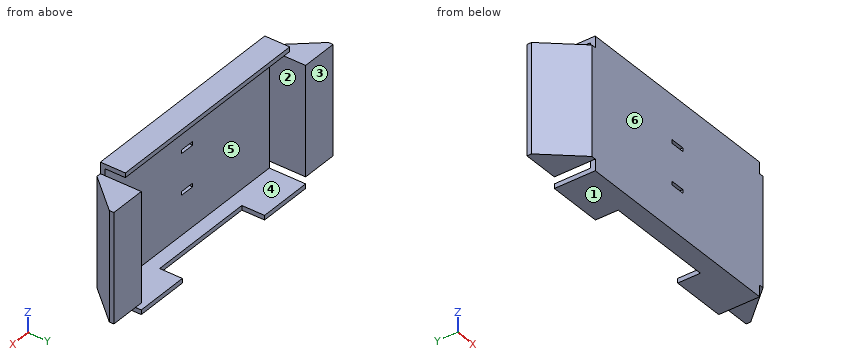
Autodesk Fusion 360 part; units mm, degrees
sketch "Sketch4" plane through (0, 0, 0) normal (0, 1, 0) x (1, 0, 0)
  line L0 (0, 0) -> (152.4, 0)
  line L1 (152.4, 0) -> (152.4, 85.725)
  line L2 (152.4, 85.725) -> (0, 85.725)
  line L3 (0, 85.725) -> (0, 0)
  dimension "d16" = 152.4
  dimension "d17" = 85.725
extrude "Extrude4" add sketch "Sketch4" along normal blind 3.175
sketch "Sketch5" plane through (0, 0, 0) normal (0, 0, 1) x (1, 0, 0)
  line L0 (0, 0) -> (152.4, 0)
  line L1 (152.4, 0) -> (152.4, 3.175)
  line L2 (152.4, 3.175) -> (0, 3.175)
  line L3 (0, 3.175) -> (0, 0)
  line L4 (0, 3.175) -> (152.4, 3.175)
  line L5 (0, 0) -> (152.4, 0)
  line L6 (0, 0) -> (0, 3.175)
  line L7 (152.4, 0) -> (152.4, 3.175)
  line L8 (152.4, 0) -> (152.4, 17.4625)
  line L9 (0, 0) -> (0, 17.4625)
  line L10 (0, 17.4625) -> (152.4, 17.4625)
  dimension "d20" = 17.4625
  dimension "d21" = 17.4625
extrude "Extrude5" add sketch "Sketch5" along normal blind 3.175
sketch "Sketch6" plane through (0, 0, -85.725) normal (0, 0, -1) x (-1, 0, 0)
  line L0 (-152.4, 0) -> (0, 0)
  line L1 (0, 0) -> (0, 3.175)
  line L2 (0, 3.175) -> (-152.4, 3.175)
  line L3 (-152.4, 3.175) -> (-152.4, 0)
  line L4 (-152.4, 3.175) -> (0, 3.175)
  line L5 (-152.4, 0) -> (-152.4, 3.175)
  line L6 (-152.4, 0) -> (0, 0)
  line L7 (0, 0) -> (0, 3.175)
  line L8 (0, 0) -> (0, 28.575)
  line L9 (0, 28.575) -> (-38.1, 28.575)
  line L10 (-38.1, 28.575) -> (-38.1, 12.7)
  line L11 (-38.1, 12.7) -> (-114.3, 12.7)
  line L12 (-114.3, 12.7) -> (-114.3, 28.575)
  line L13 (-114.3, 28.575) -> (-152.4, 28.575)
  line L14 (-152.4, 28.575) -> (-152.4, 0)
  dimension "d24" = 28.575
  dimension "d25" = 38.1
  dimension "d26" = 15.875
  dimension "d27" = 76.2
  dimension "d28" = 15.875
  dimension "d29" = 38.1
extrude "Extrude6" add sketch "Sketch6" along normal blind 3.175
sketch "Sketch7" plane through (0, 0, 0) normal (-1, 0, 0) x (0, 0, 1)
  line L0 (-88.9, 0) -> (3.175, 0)
  line L1 (3.175, 0) -> (3.175, 17.4625)
  line L2 (3.175, 17.4625) -> (0, 17.4625)
  line L3 (0, 17.4625) -> (0, 3.175)
  line L4 (0, 3.175) -> (-85.725, 3.175)
  line L5 (-85.725, 3.175) -> (-85.725, 28.575)
  line L6 (-85.725, 28.575) -> (-88.9, 28.575)
  line L7 (-88.9, 28.575) -> (-88.9, 0)
  line L8 (-85.725, 3.175) -> (-85.725, 28.575)
  line L9 (-85.725, 28.575) -> (-88.9, 28.575)
  line L10 (-88.9, 0) -> (-88.9, 28.575)
  line L11 (-85.725, 3.175) -> (0, 3.175)
  line L12 (0, 3.175) -> (0, 17.4625)
  line L13 (0, 17.4625) -> (3.175, 17.4625)
  line L14 (3.175, 17.4625) -> (3.175, 0)
  line L15 (-88.9, 0) -> (3.175, 0)
  line L16 (-85.725, 3.175) -> (-80.9625, 3.175) construction
  line L17 (0, 3.175) -> (-4.7625, 3.175) construction
  line L18 (-80.9625, 0) -> (-80.9625, 28.575)
  line L19 (-4.7625, 0) -> (-4.7625, 28.575)
  line L20 (-80.9625, 28.575) -> (-4.7625, 28.575)
  dimension "d35" = 4.7625
  dimension "d36" = 4.7625
  dimension "d37" = 28.575
  dimension "d38" = 28.575
  dimension "d39" = 76.2
extrude "Extrude7" add sketch "Sketch7" along normal blind 3.175 contours L0 L4 L11 L15 L18 L19 | L4 L11 L18 L19 L20
sketch "Sketch8" plane through (0, 28.575, 0) normal (0, 1, 0) x (-1, 0, 0)
  line L0 (0, -4.7625) -> (0, -80.9625)
  line L1 (0, -80.9625) -> (3.175, -80.9625)
  line L2 (3.175, -80.9625) -> (3.175, -4.7625)
  line L3 (3.175, -4.7625) -> (0, -4.7625)
  line L4 (0, -80.9625) -> (3.175, -80.9625)
  line L5 (0, -80.9625) -> (0, -4.7625)
  line L6 (3.175, -4.7625) -> (3.175, -80.9625)
  line L7 (0, -4.7625) -> (3.175, -4.7625)
  line L8 (0, -4.7625) -> (25.4, -4.7625)
  line L9 (0, -80.9625) -> (25.4, -80.9625)
  line L10 (25.4, -80.9625) -> (25.4, -4.7625)
  dimension "d42" = 25.4
  dimension "d43" = 25.4
  dimension "d44" = 76.2
extrude "Extrude9" add sketch "Sketch8" against normal blind 3.175 contours L2 L6 L8 L9 L10
ref_plane "WorkPlane1" through (76.2, 14.2875, -42.8625) normal (1, 0, 0) x (0, 0, -1)
mirror "Mirror1" about plane through (76.2, 14.2875, -42.8625) normal (1, 0, 0) of "Extrude7"
mirror "Mirror3" about plane through (76.2, 14.2875, -42.8625) normal (1, 0, 0) of "Extrude9"
sketch "Sketch9" plane through (0, 0, -80.9625) normal (0, 0, -1) x (-1, 0, 0)
  line L0 (-152.4, 0) -> (-152.4, 3.175)
  line L1 (-152.4, 3.175) -> (-152.4, 28.575)
  line L2 (-152.4, 28.575) -> (-177.8, 28.575)
  line L3 (-177.8, 28.575) -> (-177.8, 25.4)
  line L4 (-177.8, 25.4) -> (-155.575, 25.4)
  line L5 (-155.575, 25.4) -> (-155.575, 0)
  line L6 (-155.575, 0) -> (-152.4, 0)
  line L7 (-177.8, 25.4) -> (-155.575, 0)
extrude "Extrude10" add sketch "Sketch9" against normal up to surface (76.2 mm away) contours L4 L5 L7
mirror "Mirror4" about plane through (76.2, 14.2875, -42.8625) normal (1, 0, 0) of "Extrude10"
sketch "Sketch10" plane through (0, 3.175, 0) normal (0, 1, 0) x (-1, 0, 0)
  line L0 (0, -85.725) -> (0, -80.9625)
  line L1 (0, -80.9625) -> (0, -4.7625)
  line L2 (0, -4.7625) -> (0, 0)
  line L3 (0, 0) -> (-152.4, 0)
  line L4 (-152.4, 0) -> (-152.4, -4.7625)
  line L5 (-152.4, -4.7625) -> (-152.4, -80.9625)
  line L6 (-152.4, -80.9625) -> (-152.4, -85.725)
  line L7 (-152.4, -85.725) -> (0, -85.725)
  line L8 (0, -80.9625) -> (0, -4.7625)
  line L9 (-152.4, -85.725) -> (0, -85.725)
  line L10 (0, -85.725) -> (0, -80.9625)
  line L11 (0, -4.7625) -> (0, 0)
  line L12 (0, 0) -> (-152.4, 0)
  line L13 (-152.4, -4.7625) -> (-152.4, -80.9625)
  line L14 (-152.4, -80.9625) -> (-152.4, -85.725)
  line L15 (-152.4, 0) -> (-152.4, -4.7625)
  line L16 (0, -85.725) -> (-152.4, 0) construction
  line L17 (-152.4, -85.725) -> (0, 0) construction
  line L18 (-76.2, -42.8625) -> (-88.2955, -42.8625) construction
  line L19 (-76.2, -42.8625) -> (-64.1096, -42.8625) construction
  line L20 (-64.1096, -42.8625) -> (-64.1096, -58.3692) construction
  line L21 (-64.1096, -42.8625) -> (-64.1096, -27.3558) construction
  line L22 (-64.1096, -58.3692) -> (-88.2904, -58.3692) construction
  line L23 (-64.1096, -27.3558) -> (-88.2904, -27.3558) construction
  line L24 (-88.2904, -58.3692) -> (-88.2904, -27.3558) construction
  line L25 (-64.1096, -58.3692) -> (-71.12, -58.3692) construction
  line L26 (-88.2904, -58.3692) -> (-81.28, -58.3692) construction
  line L27 (-64.1096, -27.3558) -> (-71.12, -27.3558) construction
  line L28 (-71.12, -58.3692) -> (-71.12, -55.8292)
  line L29 (-71.12, -55.8292) -> (-81.28, -55.8292)
  line L30 (-81.28, -55.8292) -> (-81.28, -58.3692)
  line L31 (-71.12, -58.3692) -> (-81.28, -58.3692)
  line L32 (-71.12, -27.3558) -> (-71.12, -29.8958)
  line L33 (-71.12, -29.8958) -> (-81.28, -29.8958)
  line L34 (-81.28, -29.8958) -> (-81.28, -27.3558)
  line L35 (-64.1096, -27.3558) -> (-88.2904, -27.3558) construction
  line L36 (-71.12, -27.3558) -> (-81.28, -27.3558)
  point P0 (-152.4, -85.725)
  dimension "d61" = 15.5067
  dimension "d62" = 15.5067
  dimension "d63" = 24.1808
  dimension "d64" = 7.0104
  dimension "d65" = 7.0104
  dimension "d66" = 2.54
extrude "Extrude11" cut sketch "Sketch10" against normal blind 14.7066 contours L28 L29 L30 L31 | L32 L33 L34 L36
equation "d16 = 6\""
equation "d27 = 3\""
equation "d39 = 3\""
equation "d42 = 1\""
equation "d43 = 1\""
equation "d44 = 3\""
equation "d63 = ( 0.476 in + 0.476 in )"
The listing builds one solid part. Answer for the finished solid, in the listing's coordinates (mm). Face numbers are marked on the shaded views. A direction names the side the tool comes from. Coordinates: 2 decimals unless noted, no trailing zeros. Order: outer loops, then holes, each group sorted by start corner. A loop starts at its lowest first (then second) coordinate and runs counter-clockwise, first axis right, second up. Notation, with made-up numbers: (71, 15.5) -> (82, 15.5) arc R14 ccw to (82, 36.5) -> close; hole circle Ø4 at (-33, 62). An arc over 180 degrees is marked (long way). Answer in a Markdown table with one row per item. Add a question column.
Item 1: Which of the six approach directions +Z, -Z, +X, -X, +Y, -Y give full straight-line access (tool end or side, diameter ignored) to the marked faces 4, 5 and 6?
Item 2: Determine the mould class of the marked faces 1, 2 and 3 for opening direction Z: +Z half, -Z half, draft (parallel to the pull), parting line (faces both ways), or undercut.
Item 3: Find section D-D (x = 53.5). Write down the section's boundary in (y, z) (1 decimal), then the cut area to 3 significant figures.
Item 4: Find section C-C (z = -48). Write down the section's boundary in (x, y) (3 decimals), then the cut area to 3 significant figures.
Item 5: Each of these flat-tipped pins is pushed along its axis until it touches: P1, Ø3.5, axis at x = 60.5, z = 1, coming from the +Y side; P2, Ø6, axis at y = 12.5, z = -21, coming from the +X side; P3, Ø4, axis at y = 13, z = -1.5, coming from the -X side; P4, Ø8, axis at x = 72, y = 22.5, coming from the +Z side. Where does it stop, or does it pass through?
Item 6: Find section A-A (y = 15.5). Write down the section's boundary in (x, z) (1 decimal).
Item 7: Find the intervals of material crossed by L1, parallel to X at y = 25.5, z = -64.5; L2, parallel to Z at x = 76, y = 2.75 (3 decimals); L3, parallel to Z at x = 88.5, y = 11.5 (3 decimals), in increasing order. Write a range as from..to.
Item 8: Find section B-B (x = 21.5). Write down the section's boundary in (y, z) (1 decimal), then the cut area to 3 significant figures.
Result set:
| question | item | result |
|---|---|---|
| 1 | face 4 | +X, -X, +Y |
| 1 | face 5 | +Y |
| 1 | face 6 | +Z, -Z, +X, -X, -Y |
| 2 | face 1 | -Z half |
| 2 | face 2 | undercut |
| 2 | face 3 | draft |
| 3 | outline | (0, -88.9) -> (12.7, -88.9) -> (12.7, -85.7) -> (3.2, -85.7) -> (3.2, 0) -> (17.5, 0) -> (17.5, 3.2) -> (0, 3.2) -> close |
| 3 | area | 368 mm² |
| 4 | outline | (-25.4, 25.4) -> (-3.175, 0) -> (155.575, 0) -> (177.8, 25.4) -> (177.8, 28.575) -> (152.4, 28.575) -> (152.4, 3.175) -> (0, 3.175) -> (0, 28.575) -> (-25.4, 28.575) -> close |
| 4 | area | 1,370 mm² |
| 5 | P1 | stops at y = 17.46 |
| 5 | P2 | stops at x = 169.14 |
| 5 | P3 | stops at x = 0 |
| 5 | P4 | passes through |
| 6 | outline | (-16.7, -81) -> (0, -81) -> (0, -4.8) -> (-16.7, -4.8) -> close; (0, -88.9) -> (38.1, -88.9) -> (38.1, -85.7) -> (0, -85.7) -> close; (0, 0) -> (152.4, 0) -> (152.4, 3.2) -> (0, 3.2) -> close; (114.3, -88.9) -> (152.4, -88.9) -> (152.4, -85.7) -> (114.3, -85.7) -> close; (152.4, -81) -> (169.1, -81) -> (169.1, -4.8) -> (152.4, -4.8) -> close |
| 7 | L1 | x = -25.4..0, 152.4..177.8 |
| 7 | L2 | z = -88.9..-58.369, -55.829..-29.896, -27.356..3.175 |
| 7 | L3 | z = -88.9..-85.725, 0..3.175 |
| 8 | outline | (0, -88.9) -> (28.6, -88.9) -> (28.6, -85.7) -> (3.2, -85.7) -> (3.2, 0) -> (17.5, 0) -> (17.5, 3.2) -> (0, 3.2) -> close |
| 8 | area | 418 mm² |
